```python
from build123d import *

# Parameters (mm, degrees)
SKETCH3_R           = 16
BOSS_EXTRUDE1_DEPTH = 80
SKETCH4_R           = 36
BOSS_EXTRUDE2_DEPTH = 38
SKETCH6_R           = 36
SKETCH6_R_2         = 16
BOSS_EXTRUDE3_DEPTH = 35
FILLET1_R           = 5


with BuildPart() as part:
    # Sketch3 → Boss-Extrude1 (new body)
    with BuildSketch(Plane(origin=(0, 0, 0), x_dir=(0, 0, -1), z_dir=(1, 0, 0))):
        Circle(SKETCH3_R)
    extrude(amount=BOSS_EXTRUDE1_DEPTH)

    # Sketch4 → Boss-Extrude2 (add)
    with BuildSketch(Plane(origin=(80, 0, 0), x_dir=(0, 0, -1), z_dir=(1, 0, 0))):
        Circle(SKETCH4_R)
    extrude(amount=BOSS_EXTRUDE2_DEPTH)

    # Sketch6 → Boss-Extrude3 (add)
    with BuildSketch(Plane.ZY.offset(-80)):
        Circle(SKETCH6_R)
        Circle(SKETCH6_R_2, mode=Mode.SUBTRACT)
    extrude(amount=BOSS_EXTRUDE3_DEPTH)

    # Fillet1
    fillet1_edges = [part.edges().sort_by_distance(p)[0] for p in [
        (45, 0, 16),
        (0, 0, 16),
    ]]
    fillet(fillet1_edges, radius=FILLET1_R)


solid = part.part
```
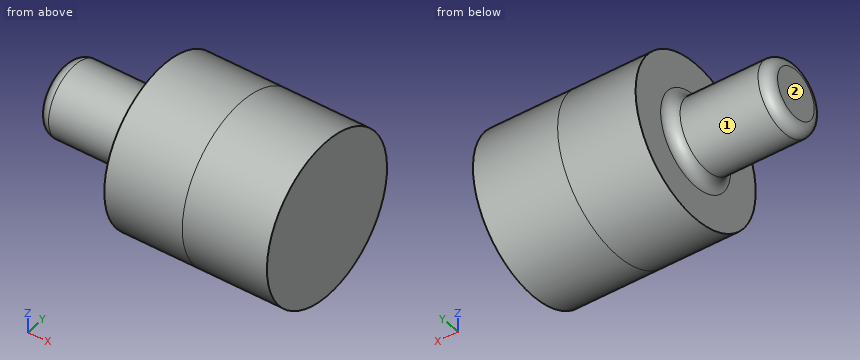
Could you check a few things on this model? Use its own coordinates, in mm. Face numbers are marked on the shaded views. A direction names the side the tool comes from. Coordinates: 2 decimals unless noted, no trailing zeros. Loops run counter-clockwise (first coordinate to the right, second up) from the corner with the lowest first, then second, coordinate; pieces in that order, holes last.
1) Imagine slicing it at A-A (y = 0). List the corners of the cut face in (x, z) for me, and give its area (3 significant figures).
Reported:
outline: (0, -11) arc R5 ccw to (5, -16) - (40, -16) arc R5 cw to (45, -21) - (45, -36) - (118, -36) - (118, 36) - (45, 36) - (45, 21) arc R5 cw to (40, 16) - (5, 16) arc R5 ccw to (0, 11) - close
area: 6,700 mm2
2) Which directions (+Z, -Z, +X, -X, +Y, -Y) give clear straight access to the entire face, cutting with the end or side of a thin tool? Please do the marked faces 1 and 2.
Reported:
face 1: -X
face 2: +Z, -Z, -X, +Y, -Y
3) Imagine slicing it at C-C (x = 26.5). List the corners of the cut face in (y, z) for me.
Reported:
outline: circle Ø32 at (0, 0)
4) Imagine slicing it at D-D (y = -26). List the corners of the cut face in (x, z) for me, and give its area (3 significant figures).
Reported:
outline: (45, -24.9) - (118, -24.9) - (118, 24.9) - (45, 24.9) - close
area: 3,640 mm2
5) Please list where these lines run through material, in increasing order: line 1 along X through (y, z) = (23, -10); line 2 along Z through (x, y) = (69, -18); line 3 along Z through (x, y) = (80, -24.5).
Reported:
line 1: x = 45 to 118
line 2: z = -31.18 to 31.18
line 3: z = -26.38 to 26.38
6) Will these pins go through, and if not, where does the flat tip stop? pin 1 Ø3 at (x, z) = (78, -23.5) entering from -Y; pin 2 Ø10 at (x, y) = (80, -19.5) entering from -Z; pin 3 Ø1.5 at (y, z) = (25, -6) entering from -X.
Reported:
pin 1: stops at y = -28.5
pin 2: stops at z = -32.95
pin 3: stops at x = 45
